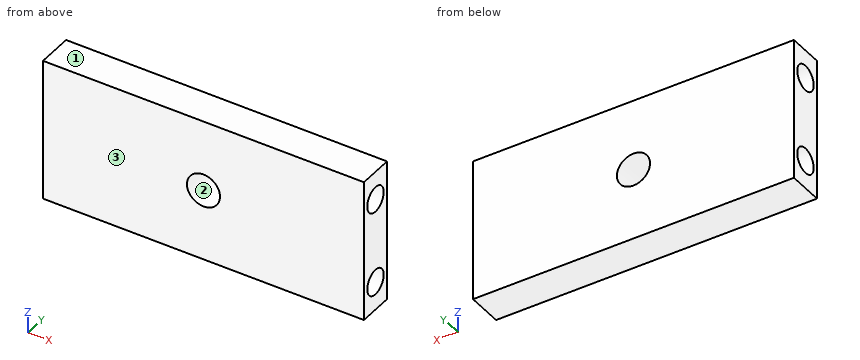
from build123d import *

# Parameters (mm, degrees)
SKETCH1_W                 = 12.7
SKETCH1_H                 = 3.175
BOSS_EXTRUDE1_DEPTH       = 28.575
F_4_CLEARANCE_HOLE1_D     = 2.9464
F_4_CLEARANCE_HOLE1_DEPTH = 3.302
F_4_CLEARANCE_HOLE1_TIP   = 0.885187864
F_4_40_TAPPED_HOLE1_D     = 2.2606
F_4_40_TAPPED_HOLE1_DEPTH = 7.62
F_4_40_TAPPED_HOLE1_TIP   = 0.679152758
F_4_40_TAPPED_HOLE2_D     = 2.2606
F_4_40_TAPPED_HOLE2_DEPTH = 7.62
F_4_40_TAPPED_HOLE2_TIP   = 0.679152758


with BuildPart() as part:
    # Sketch1 → Boss-Extrude1 (new body)
    with BuildSketch(Plane(origin=(0, 0, 0), x_dir=(0, 0, -1), z_dir=(1, 0, 0))):
        Rectangle(SKETCH1_W, SKETCH1_H)
    extrude(amount=BOSS_EXTRUDE1_DEPTH)

    # #4 Clearance Hole1
    with Locations(Plane(origin=(0, 1.5875, 0), x_dir=(1, 0, 0), z_dir=(0, 1, 0))):
        with Locations((14.2875, 0)):
            Hole(F_4_CLEARANCE_HOLE1_D / 2, depth=F_4_CLEARANCE_HOLE1_DEPTH)
            with Locations((0, 0, -(F_4_CLEARANCE_HOLE1_DEPTH + F_4_CLEARANCE_HOLE1_TIP / 2))):  # 118° drill point
                Cone(0, F_4_CLEARANCE_HOLE1_D / 2, F_4_CLEARANCE_HOLE1_TIP, mode=Mode.SUBTRACT)

    # #4-40 Tapped Hole1
    with Locations(Plane.ZY):
        with Locations((-3.81, 0), (3.81, 0)):
            Hole(F_4_40_TAPPED_HOLE1_D / 2, depth=F_4_40_TAPPED_HOLE1_DEPTH)
            with Locations((0, 0, -(F_4_40_TAPPED_HOLE1_DEPTH + F_4_40_TAPPED_HOLE1_TIP / 2))):  # 118° drill point
                Cone(0, F_4_40_TAPPED_HOLE1_D / 2, F_4_40_TAPPED_HOLE1_TIP, mode=Mode.SUBTRACT)

    # #4-40 Tapped Hole2
    with Locations(Plane(origin=(28.575, 0, 0), x_dir=(0, 0, -1), z_dir=(1, 0, 0))):
        with Locations((-3.81, 0), (3.81, 0)):
            Hole(F_4_40_TAPPED_HOLE2_D / 2, depth=F_4_40_TAPPED_HOLE2_DEPTH)
            with Locations((0, 0, -(F_4_40_TAPPED_HOLE2_DEPTH + F_4_40_TAPPED_HOLE2_TIP / 2))):  # 118° drill point
                Cone(0, F_4_40_TAPPED_HOLE2_D / 2, F_4_40_TAPPED_HOLE2_TIP, mode=Mode.SUBTRACT)


solid = part.part
Input: part model. Units: mm. Frame: model coordinates. Face numbers are marked on the shaded views. Give positions to 0.01 mm unless a question says otherwise; leave off trailing zeros. Order: outer loops, then holes, each group sorted by start corner. A loop starts at its lowest first (then second) coordinate and runs counter-clockwise, first axis right, second up. Notation, with made-up numbers: (-37, 68) - (-11, 68) arc R25 ccw to (-11, 88) - close; hole circle Ø7 at (5, -37.5). An arc over 180 degrees is marked (long way). Answer as a JSON object with one key per item and string values. Group by question number.
Q1. Mould query, pull axis Z, two halves, no side actions, for the marked faces 1, 2 and 3. Classes: pulls with the +Z half, pulls with the -Z half, needs draft (parallel to the pull), parting line crosses it, or undercut.
Q2. Cut plane C-C, the plane x = 3.5. Output: boundary loops of the cut face in (y, z).
Q3. Cut plane B-B, the plane x = 14.25. Output: boundary loops of the cut face in (y, z).
Q4. Line query: probe 1 along Z at (x, y) = (22.75, 0.05); probe 2 along Z at (x, y) = (2.25, -1); probe 3 along X at (y, z) = (0.3, -0.5) (3 decimals). Output: solid intervals per line, ascending.
Q5. First-contact query: pin 1 Ø1.8 at (y, z) = (0, -3.81) entering from +X; pin 2 Ø2.5 at (x, z) = (14.29, 0) entering from -Y; pin 3 Ø1.4 at (y, z) = (0, 3.81) entering from +X. Flat tips, straight axial feed; report the tip coordinate or a pass-through.
Q6. Cut plane A-A, the plane z = 0. Output: boundary loops of the cut face in (x, y) (1 decimal), then the cut area to 3 significant figures.
Results:
{
 "1": {"face 1": "pulls with the +Z half", "face 2": "undercut", "face 3": "needs draft"},
 "2": {"outline": "(-1.59, -6.35) - (1.59, -6.35) - (1.59, 6.35) - (-1.59, 6.35) - close; hole circle Ø2.26 at (0, -3.81); hole circle Ø2.26 at (0, 3.81)"},
 "3": {"outline": "(-1.59, -6.35) - (1.59, -6.35) - (1.59, -1.47) - (-1.59, -1.47) - close; (-1.59, 1.47) - (1.59, 1.47) - (1.59, 6.35) - (-1.59, 6.35) - close"},
 "4": {"probe 1": "-6.35 to -4.94, -2.68 to 2.68, 4.94 to 6.35", "probe 2": "-6.35 to -4.34, -3.28 to 3.28, 4.34 to 6.35", "probe 3": "0 to 12.902, 15.673 to 28.575"},
 "5": {"pin 1": "x = 20.82", "pin 2": "through", "pin 3": "x = 20.7"},
 "6": {"outline": "(0, -1.6) - (12.8, -1.6) - (12.8, 1.6) - (0, 1.6) - close; (15.8, -1.6) - (28.6, -1.6) - (28.6, 1.6) - (15.8, 1.6) - close", "area": "81.4 mm^2"}
}
